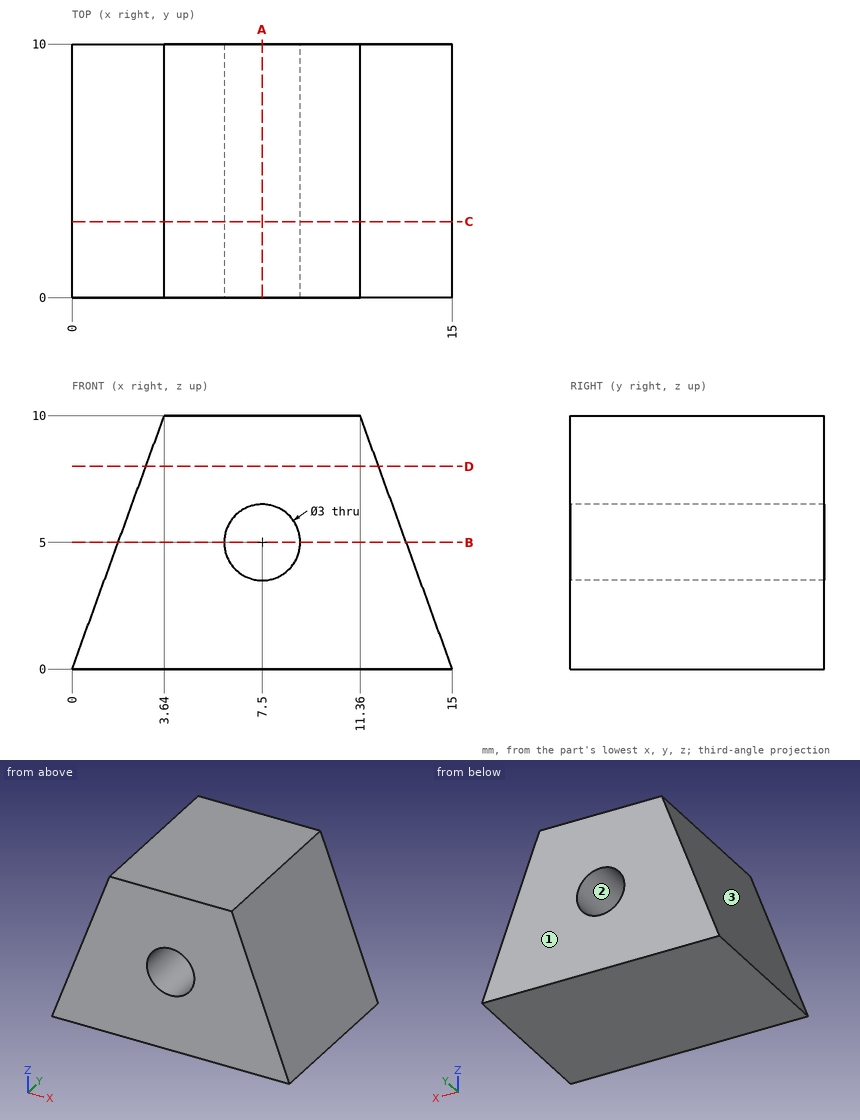
Can you work these out from the drawing? Everything is in mm from the part's minimum corner. Give positions to 0.01 mm unless a question says otherwise; leave off trailing zeros. Write each loop counter-clockwise with the first axis right and the second up, starting at its lowest first coordinate (ties: lowest second). Pieces come first, ordered by that corner, then holes. Notation, with made-up numbers: (43.5, -34.5) -> (64.5, -34.5) arc R19 cw to (64.5, -2.5) -> close; hole circle Ø6 at (5, -25.5). An arc over 180 degrees is marked (long way). Write each question's results on one line, items separated by ' | '.
Item 1: Suppose I cut it at D-D on z = 8. Write out the boundary of the cut face in (x, y).
Output:
outline: (2.91, 0) -> (12.09, 0) -> (12.09, 10) -> (2.91, 10) -> close
Item 2: Suppose I cut it at C-C on y = 3. Write out the boundary of the cut face in (x, z), plus the area to 3 significant figures.
Output:
outline: (0, 0) -> (15, 0) -> (11.36, 10) -> (3.64, 10) -> close; hole circle Ø3 at (7.5, 5) | area: 107 mm^2
Item 3: Suppose I cut it at B-B on z = 5. Write out the boundary of the cut face in (x, y), plus the area to 3 significant figures.
Output:
outline: (1.82, 0) -> (6, 0) -> (6, 10) -> (1.82, 10) -> close; (9, 0) -> (13.18, 0) -> (13.18, 10) -> (9, 10) -> close | area: 83.6 mm^2
Item 4: Suppose I cut it at A-A on x = 7.5. Write out the boundary of the cut face in (y, z), plus the area to 3 significant figures.
Output:
outline: (0, 0) -> (10, 0) -> (10, 3.5) -> (0, 3.5) -> close; (0, 6.5) -> (10, 6.5) -> (10, 10) -> (0, 10) -> close | area: 70.0 mm^2
Item 5: For pin 1 Ø5 at (x, z) = (7.5, 5) entering from -Y; pin 2 Ø4 at (y, z) = (7, 4.5) entering from -X; pin 3 Ø6 at (y, z) = (3, 7) entering from +X; pin 4 Ø6 at (y, z) = (7, 2) entering from -X, each with a flat end and sliding along its axis, tell me the tip position at first contact or that it passes through.
Output:
pin 1: stops at y = 0 | pin 2: stops at x = 0.91 | pin 3: stops at x = 13.54 | pin 4: stops at x = 0
Item 6: If I drill on L1, parallel to Z at x = 7.5, y = 4; L2, parallel to X at y = 2.25, z = 5.75; L3, parallel to X at y = 2.75, z = 4 (1 decimal), over which ranges is the centre line in solid material (lowest first)?
Output:
L1: z = 0 to 3.5, 6.5 to 10 | L2: x = 2.09 to 6.2, 8.8 to 12.91 | L3: x = 1.5 to 6.4, 8.6 to 13.5
Item 7: We'd pull the mould along X, two halves only. Please class the marked faces 1, 2 and 3: pulls with the +X half, pulls with the -X half, needs draft (parallel to the pull), parting line crosses it, or undercut.
Output:
face 1: needs draft | face 2: undercut | face 3: pulls with the -X half
